Source: CAD feature listing. Evaluate the final solid. Frame: model axes, mm. Face numbers are marked on the shaded views. A direction names the side the tool comes from. Coordinates: 2 decimals unless noted, no trailing zeros. Order: outer loops, then holes, each group sorted by start corner. A loop starts at its lowest first (then second) coordinate and runs counter-clockwise, first axis right, second up. Notation, with made-up numbers: (73, 18) -> (104, 18) arc R26 ccw to (104, 46) -> close; hole circle Ø6 at (76, 21.25). An arc over 180 degrees is marked (long way). Put each result on its own line as item: value.
from build123d import *

# Parameters (mm, degrees)
EXTRUDE_1_DEPTH     = 20
SKETCH_2_R          = 1.5
CUT_EXTRUDE_1_DEPTH = 20


with BuildPart() as part:
    # 草图1 → 凸台-拉伸1 (new body)
    with BuildSketch(Plane.XY):
        with BuildLine():
            Line((-3, 20), (-3, 10.583005244))
            ThreePointArc((-3, 10.583005244), (-11, 0), (-3, -10.583005244))
            Line((-3, -10.583005244), (-3, -50))
            Line((-3, -50), (0, -50))
            Line((0, -50), (0, -10))
            ThreePointArc((0, -10), (-10, 0), (0, 10))
            Line((0, 10), (0, 20))
            Line((0, 20), (-3, 20))
        make_face()
    extrude(amount=EXTRUDE_1_DEPTH)

    # 草图2 → 切除-拉伸1 (cut)
    with BuildSketch(Plane.ZY.offset(3)):
        with Locations((5, 15.291502622)):
            Circle(SKETCH_2_R)
        with Locations((15, 15.291502622)):
            Circle(SKETCH_2_R)
        with Locations((5, -20.291502622)):
            Circle(SKETCH_2_R)
        with Locations((15, -20.291502622)):
            Circle(SKETCH_2_R)
        with Locations((15, -40.291502622)):
            Circle(SKETCH_2_R)
        with Locations((5, -40.291502622)):
            Circle(SKETCH_2_R)
    extrude(amount=-CUT_EXTRUDE_1_DEPTH, mode=Mode.SUBTRACT)


solid = part.part
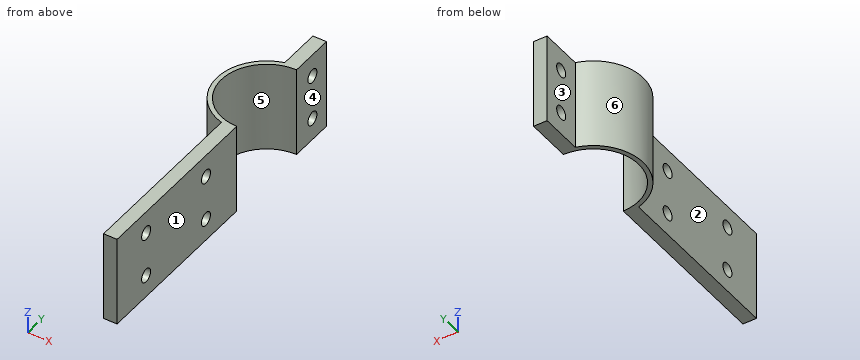
1. Cut plane A-A on z = 5. Output: boundary loops of the cut face in (x, y), plus the area to 3 significant figures.
Numbers:
outline: (-3, -50) -> (0, -50) -> (0, -41.79) -> (-3, -41.79) -> close; (-3, -38.79) -> (0, -38.79) -> (0, -21.79) -> (-3, -21.79) -> close; (-3, -18.79) -> (0, -18.79) -> (0, -10) arc R10 cw to (0, 10) -> (0, 13.79) -> (-3, 13.79) -> (-3, 10.58) arc R11 ccw to (-3, -10.58) -> close; (-3, 16.79) -> (0, 16.79) -> (0, 20) -> (-3, 20) -> close
area: 151 mm2
2. Cut plane C-C on z = 8. Output: boundary loops of the cut face in (x, y), plus the area to 3 significant figures.
Numbers:
outline: (-3, -50) -> (0, -50) -> (0, -10) arc R10 cw to (0, 10) -> (0, 20) -> (-3, 20) -> (-3, 10.58) arc R11 ccw to (-3, -10.58) -> close
area: 178 mm2
3. Pull-direction query (Y, two-part tool) for the marked faces 4, 5 and 6; classes: pulls with the +Y half, pulls with the -Y half, needs draft (parallel to the pull), parting line crosses it, or undercut.
Numbers:
face 4: needs draft
face 5: undercut
face 6: parting line crosses it
4. Cut plane B-B on x = -5.5. Output: boundary loops of the cut face in (y, z), plus the area to 3 significant figures.
Numbers:
outline: (-9.53, 0) -> (-8.35, 0) -> (-8.35, 20) -> (-9.53, 20) -> close; (8.35, 0) -> (9.53, 0) -> (9.53, 20) -> (8.35, 20) -> close
area: 47.0 mm2
5. Set-up query: the marked faces 1, 2 and 3. Return all of +Z, -Z, +X, -X, +Y, -Y with unobstructed straight access to the full face (end or side cutting, diameter ignored); none if empty.
Numbers:
face 1: +Z, -Z, +X, +Y, -Y
face 2: +Z, -Z, -X, -Y
face 3: +Z, -Z, -X, +Y
6. First-contact query: pin 1 (6 mm diameter, centred on y = 7.5, z = 15.5, fed in from +X); pin 2 (4 mm diameter, centred on y = -40.29, z = 15, fed in from -X); pin 3 (1.8 mm diameter, centred on y = -20.29, z = 5, fed in from +X). Flat tips, straight axial feed; report the tip coordinate or a pass-through.
Numbers:
pin 1: stops at x = 0
pin 2: stops at x = -3
pin 3: passes through
7. Cut plane D-D on y = 0. Output: boundary loops of the cut face in (x, z).
Numbers:
outline: (-11, 0) -> (-10, 0) -> (-10, 20) -> (-11, 20) -> close
8. Ray query, line 1 along Y through (x, z) = (-0.5, 15); line 2 along Y through (x, z) = (-2.25, 15); line 3 along Y through (x, z) = (-3.5, 1.25). Return the intervals inside material, ascending.
Numbers:
line 1: y = -50 to -41.79, -38.79 to -21.79, -18.79 to -9.99, 9.99 to 13.79, 16.79 to 20
line 2: y = -50 to -41.79, -38.79 to -21.79, -18.79 to -9.74, 9.74 to 13.79, 16.79 to 20
line 3: y = -10.43 to -9.37, 9.37 to 10.43
